CAD build for the part. Positions are in the model's coordinates, mm. Give positions to 0.01 mm unless a question says otherwise; leave off trailing zeros. Loops run counter-clockwise (first coordinate to the right, second up) from the corner with the lowest first, then second, coordinate; pieces in that order, holes last. Notation, with made-up numbers: M -1.75,9 L 7.25,9 A23 cw 7.25,19 Z; hole C 62.5,44 d6. An arc over 180 degrees is marked long. One line per question, with ' | ' between items.
```python
from build123d import *

# Parameters (mm, degrees)
SKETCH1_W           = 6.35
SKETCH1_H           = 76.2
BOSS_EXTRUDE1_DEPTH = 457.2
SKETCH2_W           = 6.35
SKETCH2_H           = 50.8
BOSS_EXTRUDE2_DEPTH = 6.35
SKETCH3_W           = 6.35
SKETCH3_H           = 12.7
CUT_EXTRUDE1_DEPTH  = 460.399570091
SKETCH4_W           = 6.35
SKETCH4_H           = 12.7
BOSS_EXTRUDE4_DEPTH = 6.35
SKETCH7_R           = 2.0955
CUT_EXTRUDE2_DEPTH  = 460.399570091
SKETCH9_R           = 2.0955
SKETCH9_W           = 25.4
SKETCH9_H           = 6.35
CUT_EXTRUDE3_DEPTH  = 6.35
CUT_EXTRUDE4_DEPTH  = 6.35


with BuildPart() as part:
    # Sketch1 → Boss-Extrude1 (new body)
    with BuildSketch(Plane.XY):
        with Locations((-41.275, 0)):
            Rectangle(SKETCH1_W, SKETCH1_H)
    extrude(amount=-BOSS_EXTRUDE1_DEPTH)

    # Sketch2 → Boss-Extrude2 (add)
    with BuildSketch(Plane(origin=(0, 38.1, 0), x_dir=(1, 0, 0), z_dir=(0, 1, 0))):
        with Locations((-41.275, 381)):
            Rectangle(SKETCH2_W, SKETCH2_H)
        with Locations((-41.275, 279.4)):
            Rectangle(SKETCH2_W, SKETCH2_H)
        with Locations((-41.275, 177.8)):
            Rectangle(SKETCH2_W, SKETCH2_H)
        with Locations((-41.275, 76.2)):
            Rectangle(SKETCH2_W, SKETCH2_H)
    extrude(amount=BOSS_EXTRUDE2_DEPTH)

    # Sketch3 → Cut-Extrude1 (cut, through all)
    with BuildSketch(Plane(origin=(-38.1, 0, 0), x_dir=(0, 0, -1), z_dir=(1, 0, 0))):
        with Locations((85.725, 19.05)):
            Rectangle(SKETCH3_W, SKETCH3_H)
        with Locations((85.725, -19.05)):
            Rectangle(SKETCH3_W, SKETCH3_H)
    extrude(amount=-CUT_EXTRUDE1_DEPTH, mode=Mode.SUBTRACT)

    # Sketch4 → Boss-Extrude4 (add)
    with BuildSketch(Plane.XY):
        with Locations((-41.275, 0)):
            Rectangle(SKETCH4_W, SKETCH4_H)
    extrude(amount=BOSS_EXTRUDE4_DEPTH)

    # Sketch7 → Cut-Extrude2 (cut, through all)
    with BuildSketch(Plane.ZY.offset(44.45)):
        with Locations((-241.3, -12.7)):
            Circle(SKETCH7_R)
        with Locations((-241.3, 12.7)):
            Circle(SKETCH7_R)
        with Locations((-437.8325, -12.7)):
            Circle(SKETCH7_R)
        with Locations((-437.8325, 12.7)):
            Circle(SKETCH7_R)
    extrude(amount=-CUT_EXTRUDE2_DEPTH, mode=Mode.SUBTRACT)

    # Sketch9 → Cut-Extrude3 (cut)
    with BuildSketch(Plane.ZY.offset(44.45)):
        with Locations((-114.880216651, 6.35)):
            Circle(SKETCH9_R)
        with Locations((-228.517018256, 6.35)):
            Circle(SKETCH9_R)
        with Locations((-254, 6.35)):
            Rectangle(SKETCH9_W, SKETCH9_H)
        with Locations((-203.2, 6.35)):
            Rectangle(SKETCH9_W, SKETCH9_H)
        with Locations((-152.4, 6.35)):
            Rectangle(SKETCH9_W, SKETCH9_H)
    extrude(amount=-CUT_EXTRUDE3_DEPTH, mode=Mode.SUBTRACT)

    # Sketch10 → Cut-Extrude4 (cut)
    with BuildSketch(Plane(origin=(-38.1, 0, 0), x_dir=(0, 0, -1), z_dir=(1, 0, 0))):
        Polygon((0, 24.548534751), (0, 20.281334751), (8.763, 20.281334751), (8.763, 17.969934751), (11.938, 17.969934751), (11.938, 20.281334751), (15.24, 20.281334751), (15.24, 24.548534751), (11.938, 24.548534751), (11.938, 26.859934751), (8.763, 26.859934751), (8.763, 24.548534751), align=None)
        Polygon((0, -20.0914), (0, -24.3586), (8.763, -24.3586), (8.763, -26.67), (11.938, -26.67), (11.938, -24.3586), (15.24, -24.3586), (15.24, -20.0914), (11.938, -20.0914), (11.938, -17.78), (8.763, -17.78), (8.763, -20.0914), align=None)
        Polygon((332.3336, 38.1), (328.0664, 38.1), (328.0664, 29.337), (325.755, 29.337), (325.755, 26.162), (328.0664, 26.162), (328.0664, 22.86), (332.3336, 22.86), (332.3336, 26.162), (334.645, 26.162), (334.645, 29.337), (332.3336, 29.337), align=None)
        Polygon((229.270305867, 38.1), (225.003105867, 38.1), (225.003105867, 29.337), (222.691705867, 29.337), (222.691705867, 26.162), (225.003105867, 26.162), (225.003105867, 22.86), (229.270305867, 22.86), (229.270305867, 26.162), (231.581705867, 26.162), (231.581705867, 29.337), (229.270305867, 29.337), align=None)
        Polygon((129.1336, 38.1), (124.8664, 38.1), (124.8664, 29.337), (122.555, 29.337), (122.555, 26.162), (124.8664, 26.162), (124.8664, 22.86), (129.1336, 22.86), (129.1336, 26.162), (131.445, 26.162), (131.445, 29.337), (129.1336, 29.337), align=None)
    extrude(amount=-CUT_EXTRUDE4_DEPTH, mode=Mode.SUBTRACT)


solid = part.part
```
Item 1: Saw through at A-A on z = -196.5. Give the cut face in (x, y) (3 decimals), and give its area (3 significant figures).
Conclusion:
outline: M -44.45,-38.1 L -38.1,-38.1 L -38.1,3.175 L -44.45,3.175 Z; M -44.45,9.525 L -38.1,9.525 L -38.1,44.45 L -44.45,44.45 Z | area: 484 mm²
Item 2: Drop flat-ended pins along their axis: P1, Ø1.9, axis at x = -42, y = 40.5, coming from the -Z side; P2, Ø3.5, axis at x = -41.5, y = 24.5, coming from the +Z side; P3, Ø3, axis at x = -40.5, z = -245, coming from the +Y side; P4, Ø2.5, axis at y = 12.7, z = -437.83, coming from the +X side. Give the stop position or say it passes through.
Conclusion:
P1: z = -406.4 | P2: z = 0 | P3: y = 38.1 | P4: through
Item 3: Saw through at B-B on x = -42. State how many separate pieces and enclosed holes the cut face has, and give its area (3 significant figures).
Conclusion:
separate pieces: 1 | enclosed holes: 11 | area: 35,100 mm²
Item 4: Drill centre lines: line 1 along Z through (x, y) = (-42, 32); line 2 along Z through (x, y) = (-38.25, 19); line 3 along Z through (x, y) = (-42, 16.5). Where is each one in solid material? Low to high. Write a range as [from, to].
Conclusion:
line 1: [-457.2, -332.33], [-328.07, -229.27], [-225, -129.13], [-124.87, 0] | line 2: [-457.2, -88.9], [-82.55, -11.94], [-8.76, 0] | line 3: [-457.2, -88.9], [-82.55, 0]
